```python
from build123d import *

# Parameters (mm, degrees)
SKETCH1_W              = 33.02
SKETCH1_H              = 13.97
DEPTH_A_DEPTH          = 6.35
ROUND_EXTRUDE_DEPTH    = 33.02
ANGLE_CUT_DEPTH        = 39.253150524
STRING_HOLE_R          = 0.762
STRING_HOLE_CUT_DEPTH  = 39.253150524
ELASTIC_HOLES_R        = 2.54
ELASTIC_HOLE_CUT_DEPTH = 39.253150524


with BuildPart() as part:
    # Sketch1 → depth a (new body)
    with BuildSketch(Plane(origin=(0, 0, 0), x_dir=(1, 0, 0), z_dir=(0, 1, 0))):
        with Locations((-16.51, 6.985)):
            Rectangle(SKETCH1_W, SKETCH1_H)
    extrude(amount=DEPTH_A_DEPTH)

    # Sketch4 → round extrude (add)
    with BuildSketch(Plane(origin=(0, 0, 0), x_dir=(0, 0, -1), z_dir=(1, 0, 0))):
        with BuildLine():
            Line((0, 6.35), (13.97, 6.35))
            ThreePointArc((13.97, 6.35), (6.985, 13.335), (0, 6.35))
        make_face()
    extrude(amount=-ROUND_EXTRUDE_DEPTH)

    # Sketch5 → angle cut (cut, through all)
    with BuildSketch(Plane.XY):
        Polygon((0, 6.35), (0, 13.335), (-6.985, 13.335), align=None)
        Polygon((-33.02, 6.35), (-33.02, 13.335), (-26.035, 13.335), align=None)
    extrude(amount=-ANGLE_CUT_DEPTH, mode=Mode.SUBTRACT)

    # string hole → string hole cut (cut, through all)
    with BuildSketch(Plane(origin=(0, 0, 0), x_dir=(0, 0, -1), z_dir=(1, 0, 0))):
        with Locations(Location((6.985, 11.684, 0), (0, 0, 270))):
            Circle(STRING_HOLE_R)
    extrude(amount=-STRING_HOLE_CUT_DEPTH, mode=Mode.SUBTRACT)

    # elastic holes → elastic hole cut (cut, through all)
    with BuildSketch(Plane(origin=(0, 0, 0), x_dir=(0, 0, -1), z_dir=(1, 0, 0))):
        with Locations((3.4925, 3.175)):
            Circle(ELASTIC_HOLES_R)
        with Locations(Location((10.4775, 3.175, 0), (0, 0, 180))):
            Circle(ELASTIC_HOLES_R)
    extrude(amount=-ELASTIC_HOLE_CUT_DEPTH, mode=Mode.SUBTRACT)


solid = part.part
```
Build history of the part. All positions in model axes, mm. Coordinates: 2 decimals unless noted, no trailing zeros. Order: outer loops, then holes, each group sorted by start corner. A loop starts at its lowest first (then second) coordinate and runs counter-clockwise, first axis right, second up. Notation, with made-up numbers: M 68.5,-6.5 L 123.5,-6.5 A7 ccw 123.5,-2.5 Z; hole C 56.5,64 d5. An arc over 180 degrees is marked long. One line per question, with ' | ' between items. Start each with the question number.
1. Mould opens along Z. For faces 1 (the face through (-17, 3, 0)), 2 (the face through (-16.3, 1.6, -1.5)), 3 (the face through (-16.279, 13.333, -7.139)) say: +Z half, -Z half, draft (parallel to the pull), parting line (faces both ways), or undercut.
2. Wall check: line 1 along Z through (x, y) = (-13.5, 1.5); line 2 along Z through (x, y) = (-22, 3.25); line 3 along Y through (x, z) = (-28, -3). Give the ranges that are in metal, low to high. Write a range as [from, to].
3. Cut at A-A (z = -2.25). Write the cut outline in (x, y), plus the area to 3 significant figures.
4. Cut at B-B (x = -19.5). Count the separate pieces of the cut face and the enclosed holes in it, plus the area to 3 significant figures.
5. Flat gauge pins, fed straight in: P1, Ø4.5, axis at y = 3.18, z = -10.48, coming from the -X side; P2, Ø2.5, axis at y = 11.684, z = -6.985, coming from the +X side. Where does each tip first touch, or does it go through?
6. Cut at D-D (y = 9.5). Write the cut outline in (x, z), plus the area to 3 significant figures.
The answers:
1) face 1: +Z half | face 2: undercut | face 3: parting line
2) line 1: z = [-13.97, -12.39], [-8.57, -5.4], [-1.58, 0] | line 2: z = [-13.97, -13.02], [-7.94, -6.03], [-0.95, 0] | line 3: y = [0, 0.68], [5.67, 11.37]
3) outline: M -33.02,0 L 0,0 L 0,0.96 L -33.02,0.96 Z; M -33.02,5.39 L 0,5.39 L 0,6.35 L -5.14,11.49 L -27.88,11.49 L -33.02,6.35 Z | area: 207 mm2
4) separate pieces: 1 | enclosed holes: 3 | area: 123 mm2
5) P1: passes through | P2: stops at x = -4.08
6) outline: M -29.87,-13.22 L -3.15,-13.22 L -3.15,-0.75 L -29.87,-0.75 Z | area: 333 mm2
